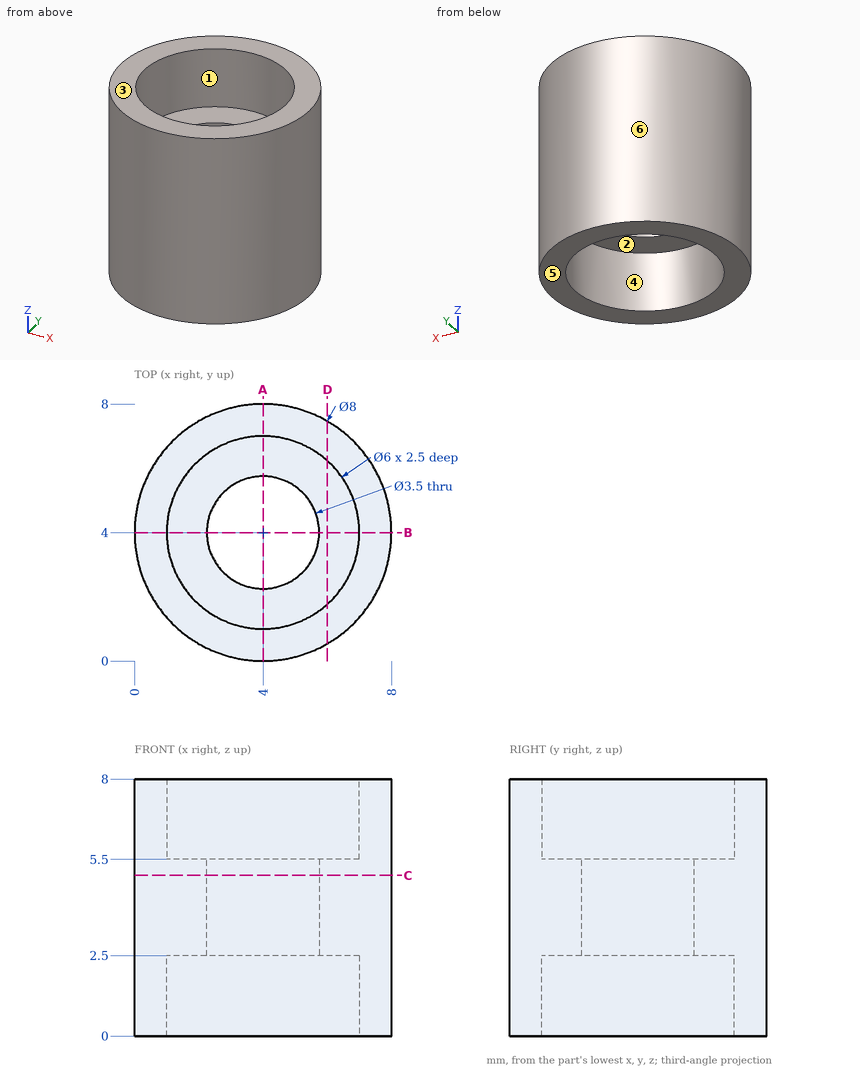
Could you check a few things on this drawing? It's one solid part, dimensions in mm from its lowest x, y, z. A direction names the side the tool comes from. Give positions to 0.01 mm unless a question says otherwise; leave off trailing zeros. Loops run counter-clockwise (first coordinate to the right, second up) from the corner with the lowest first, then second, coordinate; pieces in that order, holes last. Notation, with made-up numbers: M 23,56.25 L 65,56.25 A16 cw 65,87.25 Z; hole C -31.75,-6 d9. An arc over 180 degrees is marked long. Answer as a JSON object with one key per item and string values.
Q1. For P1, Ø1.5, axis at x = 1, z = 6, coming from the +Y side; P2, Ø3, axis at x = 3, y = 4.5, coming from the +Z side; P3, Ø2, axis at x = 4, y = 4, coming from the -Z side; P4, Ø1.5, axis at y = 1, z = 1.5, coming from the -X side, each with a flat end and sliding along its axis, tell me the tip position at first contact or that it passes through.
Values found:
{"P1": "stops at y = 7.31", "P2": "stops at z = 5.5", "P3": "passes through", "P4": "stops at x = 0.69"}
Q2. If I drill on probe 1 along Y at (x, z) = (4, 1.6); probe 2 along Y at (x, z) = (4, 4.65); probe 3 along Z at (x, y) = (5.5, 5), over which ranges is the centre line in solid material (lowest first)? Write a range as [from, to].
Values found:
{"probe 1": "y = [0, 1], [7, 8]", "probe 2": "y = [0, 2.25], [5.75, 8]", "probe 3": "z = [2.5, 5.5]"}
Q3. Suppose I cut it at D-D, the plane x = 6. List the corners of the cut face in (y, z) for me.
Values found:
{"outline": "M 0.54,0 L 1.76,0 L 1.76,2.5 L 6.24,2.5 L 6.24,0 L 7.46,0 L 7.46,8 L 6.24,8 L 6.24,5.5 L 1.76,5.5 L 1.76,8 L 0.54,8 Z"}
Q4. For the marked faces 1, 2 and 3, which set-ups out of +Z, -Z, +X, -X, +Y, -Y let a thin tool reach every point of the face, with its end or its side?
Values found:
{"face 1": "+Z", "face 2": "-Z", "face 3": "+Z, +X, -X, +Y, -Y"}
Q5. Suppose I cut it at C-C, the plane z = 5. List the corners of the cut face in (x, y) for me, plus the area to 3 significant figures.
Values found:
{"outline": "C 4,4 d8; hole C 4,4 d3.5", "area": "40.6 mm²"}
Q6. If we mould it in two halves opening along X, with no side actions, what happens to the marked faces 4, 5 and 6? For each: pulls with the +X half, pulls with the -X half, needs draft (parallel to the pull), parting line crosses it, or undercut.
Values found:
{"face 4": "undercut", "face 5": "needs draft", "face 6": "parting line crosses it"}
Q7. Suppose I cut it at A-A, the plane x = 4. List the corners of the cut face in (y, z) for me.
Values found:
{"outline": "M 0,0 L 1,0 L 1,2.5 L 2.25,2.5 L 2.25,5.5 L 1,5.5 L 1,8 L 0,8 Z; M 5.75,2.5 L 7,2.5 L 7,0 L 8,0 L 8,8 L 7,8 L 7,5.5 L 5.75,5.5 Z"}
